Read the model definition and answer for the solid it produces. Units are mm, in the model's axes. A direction names the side the tool comes from. Give positions to 0.01 mm unless a question says otherwise; leave off trailing zeros. Order: outer loops, then holes, each group sorted by start corner. A loop starts at its lowest first (then second) coordinate and runs counter-clockwise, first axis right, second up.
```python
from build123d import *

# Parameters (mm, degrees)
ESQUISSE1_W        = 150
ESQUISSE1_H        = 75
ESQUISSE1_R        = 2.25
ESQUISSE1_W_2      = 6
ESQUISSE1_H_2      = 3
ESQUISSE1_W_3      = 17
ESQUISSE1_H_3      = 7
BOSS_EXTRU_1_DEPTH = 5


with BuildPart() as part:
    # Esquisse1 → Boss.-Extru.1 (new body)
    with BuildSketch(Plane.XY):
        with Locations((75, -37.5)):
            Rectangle(ESQUISSE1_W, ESQUISSE1_H)
        with Locations((8.5, -64)):
            Circle(ESQUISSE1_R, mode=Mode.SUBTRACT)
        with Locations((141.5, -64)):
            Circle(ESQUISSE1_R, mode=Mode.SUBTRACT)
        with Locations((57, -14)):
            Circle(ESQUISSE1_R, mode=Mode.SUBTRACT)
        with Locations((93, -14)):
            Circle(ESQUISSE1_R, mode=Mode.SUBTRACT)
        with Locations((93, -50)):
            Circle(ESQUISSE1_R, mode=Mode.SUBTRACT)
        with Locations((57, -50)):
            Circle(ESQUISSE1_R, mode=Mode.SUBTRACT)
        with Locations((75, -14)):
            Circle(ESQUISSE1_R, mode=Mode.SUBTRACT)
        with Locations((75, -50)):
            Circle(ESQUISSE1_R, mode=Mode.SUBTRACT)
        with Locations((8.5, -59.5)):
            Rectangle(ESQUISSE1_W_2, ESQUISSE1_H_2, mode=Mode.SUBTRACT)
        with Locations((8.5, -73.4)):
            Rectangle(ESQUISSE1_W_2, ESQUISSE1_H_2, mode=Mode.SUBTRACT)
        with Locations((141.5, -59.5)):
            Rectangle(ESQUISSE1_W_2, ESQUISSE1_H_2, mode=Mode.SUBTRACT)
        with Locations((141.5, -73.4)):
            Rectangle(ESQUISSE1_W_2, ESQUISSE1_H_2, mode=Mode.SUBTRACT)
        with Locations((33.5, -49.5)):
            Rectangle(ESQUISSE1_W_3, ESQUISSE1_H_3, mode=Mode.SUBTRACT)
        with Locations((116.5, -49.5)):
            Rectangle(ESQUISSE1_W_3, ESQUISSE1_H_3, mode=Mode.SUBTRACT)
    extrude(amount=BOSS_EXTRU_1_DEPTH)


solid = part.part
```
1) The part is cut by section A-A on x = 75. Determine the outline of the cut face in (y, z), and give its area (3 significant figures).
Final values:
outline: (-75, 0) - (-52.25, 0) - (-52.25, 5) - (-75, 5) - close; (-47.75, 0) - (-16.25, 0) - (-16.25, 5) - (-47.75, 5) - close; (-11.75, 0) - (0, 0) - (0, 5) - (-11.75, 5) - close
area: 330 mm2
2) For a pull along X with two mould halves and no side action, classify faces 1 (the face through (144.5, -73, 2)), 2 (the face through (150, -38, 2)), 3 (the face through (74, -75, 2)) as released by +X, released by -X, zero draft, split by the parting line, or undercut.
Final values:
face 1: undercut
face 2: released by +X
face 3: zero draft
3) The part is cut by section D-D on x = 27.5. Determine the outline of the cut face in (y, z).
Final values:
outline: (-75, 0) - (-53, 0) - (-53, 5) - (-75, 5) - close; (-46, 0) - (0, 0) - (0, 5) - (-46, 5) - close
4) The part is cut by section C-C on y = -14. Determine the outline of the cut face in (x, z), and give its area (4 significant figures).
Final values:
outline: (0, 0) - (54.75, 0) - (54.75, 5) - (0, 5) - close; (59.25, 0) - (72.75, 0) - (72.75, 5) - (59.25, 5) - close; (77.25, 0) - (90.75, 0) - (90.75, 5) - (77.25, 5) - close; (95.25, 0) - (150, 0) - (150, 5) - (95.25, 5) - close
area: 682.5 mm2
5) Consider L1, parallel to X at y = -46.5, z = 0.45; L2, parallel to Y at x = 75, z = 2.9; L3, parallel to Y at x = 118.5, z = 2. Determine where each line is inside the solid, lowest interval first.
Final values:
L1: x = 0 to 25, 42 to 108, 125 to 150
L2: y = -75 to -52.25, -47.75 to -16.25, -11.75 to 0
L3: y = -75 to -53, -46 to 0
6) The part is cut by section B-B on x = 141.5. Determine the outline of the cut face in (y, z), and give its area (4 significant figures).
Final values:
outline: (-75, 0) - (-74.9, 0) - (-74.9, 5) - (-75, 5) - close; (-71.9, 0) - (-66.25, 0) - (-66.25, 5) - (-71.9, 5) - close; (-61.75, 0) - (-61, 0) - (-61, 5) - (-61.75, 5) - close; (-58, 0) - (0, 0) - (0, 5) - (-58, 5) - close
area: 322.5 mm2
7) Given pin 1 (2.5 mm diameter, centred on x = 113.5, z = 1.5, fed in from +Y), flat-ended and moving along its own axis, determine where the tip first touches the part or whether it passes through.
Final values:
pin 1: stops at y = 0
8) A tool of negligible diameter and unlimited length cuts with its end or side. For faces 4 (the face through (74, -37, 0)), 5 (the face through (5.5, -60, 2)), from which of +Z, -Z, +X, -X, +Y, -Y can it reach the whole face along a straight path? Write none if from no direction.
Final values:
face 4: -Z, +X, -X, +Y, -Y
face 5: +Z, -Z
